Can you work these out from the model? Positions are in its coordinate system, mm. Face numbers are marked on the shaded views. A direction names the side the tool comes from. Give positions to 0.01 mm unless a question says otherwise; leave off trailing zeros. Loops run counter-clockwise (first coordinate to the right, second up) from the corner with the lowest first, then second, coordinate; pieces in that order, holes last. Notation, with made-up numbers: (17, 60.25) - (55, 60.25) arc R20 cw to (55, 94.25) - close; hole circle Ø8 at (4.25, 79.25). An arc over 180 degrees is marked (long way). Answer as a JSON object with one key per item and string values.
```python
from build123d import *

# Parameters (mm, degrees)
F0_W     = 9
F0_H     = 19
F1_DEPTH = 11
F3_R     = 2
F4_DEPTH = 11
F6_W     = 4.6
F6_H     = 3.6
F6_H_2   = 2.2
F7_DEPTH = 8.9
F8_W     = 9.0002920479
F8_H     = 4
F9_DEPTH = 5
F10_R    = 1.5


with BuildPart() as f1:
    # F0 (on Top) → F1 (new body)
    with BuildSketch(Plane.XY):
        Rectangle(F0_W, F0_H)
    extrude(amount=F1_DEPTH)

    # F3 (on offset) → F4 (cut)
    with BuildSketch(Plane(origin=(0, 0, 0), x_dir=(1, 0, 0), z_dir=(0, 0, -1))):
        with Locations((0, 5.0686830655)):
            Circle(F3_R)
    extrude(amount=-F4_DEPTH, mode=Mode.SUBTRACT)

    # F6 (on offset) → F7 (cut)
    with BuildSketch(Plane.XY.offset(11)):
        with Locations((0, 3.3313169345)):
            Rectangle(F6_W, F6_H)
        with Locations((0, 6.2313169345)):
            Rectangle(F6_W, F6_H_2)
        with Locations((0, 0.4313169345)):
            Rectangle(F6_W, F6_H_2)
    extrude(amount=-F7_DEPTH, mode=Mode.SUBTRACT)

    # F8 (on offset) → F9 (cut)
    with BuildSketch(Plane.XY.offset(11)):
        with Locations((0, 3.3313169345)):
            Rectangle(F8_W, F8_H)
    extrude(amount=-F9_DEPTH, mode=Mode.SUBTRACT)

    # F10
    f10_edges = [f1.edges().sort_by_distance(p)[0] for p in [
        (4.5, 9.5, 5.5),
        (-4.5, 9.5, 5.5),
        (4.5, -9.5, 5.5),
        (-4.5, -9.5, 5.5),
    ]]
    fillet(f10_edges, radius=F10_R)


solid = f1.part
```
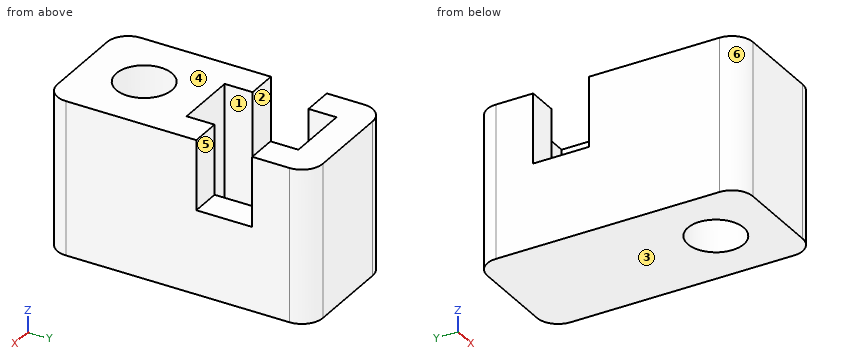
1) Which directions (+Z, -Z, +X, -X, +Y, -Y) give clear straight access to the entire face, cutting with the end or side of a thin tool? Please do the marked faces 1, 2 and 3.
Check sheet entries:
{"face 1": "+Z", "face 2": "+Z, +X, -X", "face 3": "-Z, +X, -X, +Y, -Y"}
2) If we mould it in two halves opening along Y, with no side actions, what happens to the marked faces 4, 5 and 6? For each: released by +Y, released by -Y, zero draft, split by the parting line, or undercut.
Check sheet entries:
{"face 4": "zero draft", "face 5": "undercut", "face 6": "released by -Y"}
3) I need wall thicknesses on L1, parallel to Y at x = 0, z = 8; L2, parallel to X at y = 1, z = 9.75; L3, parallel to Y at x = -0.75, z = 10. Which ranges of each line are inside material? Lowest first, please.
Check sheet entries:
{"L1": "-9.5 to -7.07, -3.07 to -0.67, 7.33 to 9.5", "L2": "-4.5 to -2.3, 2.3 to 4.5", "L3": "-9.5 to -6.92, -3.21 to -0.67, 7.33 to 9.5"}
4) I'm going to push flat-ended pins straight in: P1, Ø0.7, axis at x = 3.5, z = 8, coming from the +Y side; P2, Ø2.5, axis at x = -0.5, y = 1.5, coming from the +Z side; P3, Ø1.8, axis at x = 3.5, y = 2.5, coming from the +Z side. Where does each tip first touch, or does it pass through?
Check sheet entries:
{"P1": "y = 9.49", "P2": "z = 2.1", "P3": "z = 6"}
5) Imagine slicing it at C-C on y = 5.75. Write out the boundary of the cut face in (x, z).
Check sheet entries:
{"outline": "(-4.5, 0) - (4.5, 0) - (4.5, 11) - (2.3, 11) - (2.3, 2.1) - (-2.3, 2.1) - (-2.3, 11) - (-4.5, 11) - close"}
6) Imagine slicing it at A-A on x = 0. Write out the boundary of the cut face in (y, z).
Check sheet entries:
{"outline": "(-9.5, 0) - (-7.07, 0) - (-7.07, 11) - (-9.5, 11) - close; (-3.07, 0) - (9.5, 0) - (9.5, 11) - (7.33, 11) - (7.33, 2.1) - (-0.67, 2.1) - (-0.67, 11) - (-3.07, 11) - close"}
7) Imagine slicing it at B-B on z = 8.25. Write out the boundary of the cut face in (x, y).
Check sheet entries:
{"outline": "(-4.5, -8) arc R1.5 ccw to (-3, -9.5) - (3, -9.5) arc R1.5 ccw to (4.5, -8) - (4.5, 1.33) - (2.3, 1.33) - (2.3, -0.67) - (-2.3, -0.67) - (-2.3, 1.33) - (-4.5, 1.33) - close; (-4.5, 5.33) - (-2.3, 5.33) - (-2.3, 7.33) - (2.3, 7.33) - (2.3, 5.33) - (4.5, 5.33) - (4.5, 8) arc R1.5 ccw to (3, 9.5) - (-3, 9.5) arc R1.5 ccw to (-4.5, 8) - close; hole circle Ø4 at (0, -5.07)"}
8) Imagine slicing it at D-D on z = 2.75. Write out the boundary of the cut face in (x, y).
Check sheet entries:
{"outline": "(-4.5, -8) arc R1.5 ccw to (-3, -9.5) - (3, -9.5) arc R1.5 ccw to (4.5, -8) - (4.5, 8) arc R1.5 ccw to (3, 9.5) - (-3, 9.5) arc R1.5 ccw to (-4.5, 8) - close; hole (-2.3, -0.67) - (2.3, -0.67) - (2.3, 7.33) - (-2.3, 7.33) - close; hole circle Ø4 at (0, -5.07)"}
